Verification items for the finished model (mm, model axes). A direction names the side the tool comes from. Coordinates: 2 decimals unless noted, no trailing zeros. Write each loop counter-clockwise with the first axis right and the second up, starting at its lowest first coordinate (ties: lowest second). Pieces come first, ordered by that corner, then holes. Notation, with made-up numbers: (4.5, 57.5) -> (59.5, 57.5) arc R14 cw to (59.5, 78.5) -> close; hole circle Ø1 at (48, 68.25). An arc over 180 degrees is marked (long way). Answer in a Markdown table with one row per item.
```python
from build123d import *

# Parameters (mm, degrees)
F1_DEPTH      = 300
F1_DEPTH_BACK = 300


with BuildPart() as f1:
    # F0 (on Right) → F1 (new body, two sides)
    with BuildSketch(Plane.YZ) as f1_sk:
        with BuildLine():
            Line((110.183008, 157.357644), (5.9717, 8.528471))
            ThreePointArc((5.9717, 8.528471), (-1.176369, 2.259783), (-10.411341, 0))
            Line((-10.411341, 0), (-160.408616, 0))
            Line((-160.408616, 0), (-160.411341, -4))
            Line((-160.411341, -4), (-10.411341, -4))
            ThreePointArc((-10.411341, -4), (0.670626, -1.28826), (9.248308, 6.234166))
            Line((9.248308, 6.234166), (113.459616, 155.063338))
            ThreePointArc((113.459616, 155.063338), (147.770346, 185.15304), (192.098213, 196))
            Line((192.098213, 196), (231.673377, 196))
            ThreePointArc((231.673377, 196), (242.48282, 191.796437), (247.612492, 181.394492))
            Line((247.612492, 181.394492), (261.915687, 17.908216))
            ThreePointArc((261.915687, 17.908216), (269.610202, 2.305292), (285.824377, -4.000046))
            Line((285.824377, -4.000046), (339.588671, -4.000007))
            ThreePointArc((339.588671, -4.000007), (350.670628, -1.288263), (359.248303, 6.234158))
            Line((359.248303, 6.234158), (463.459616, 155.063338))
            ThreePointArc((463.459616, 155.063338), (497.770346, 185.15304), (542.098213, 196))
            Line((542.098213, 196), (581.673377, 196))
            ThreePointArc((581.673377, 196), (591.80723, 192.05916), (596.616297, 182.307336))
            Line((596.616297, 182.307336), (610.919489, 18.821106))
            ThreePointArc((610.919489, 18.821106), (618.613997, 3.218188), (634.828161, -3.087156))
            Line((634.828161, -3.087156), (688.592464, -3.087156))
            ThreePointArc((688.592464, -3.087156), (699.674431, -0.375416), (708.252113, 7.14701))
            Line((708.252113, 7.14701), (812.463422, 155.976182))
            ThreePointArc((812.463422, 155.976182), (846.774151, 186.065884), (891.102018, 196.912844))
            Line((891.102018, 196.912844), (930.677182, 196.912844))
            ThreePointArc((930.677182, 196.912844), (940.810305, 192.972673), (945.61993, 183.222154))
            Line((945.61993, 183.222154), (961.032927, -3.087156))
            Line((961.032927, -3.087156), (965.046592, -3.087156))
            Line((965.046592, -3.087156), (949.605558, 183.561051))
            ThreePointArc((949.605558, 183.561051), (943.516264, 195.918485), (930.677182, 200.912844))
            Line((930.677182, 200.912844), (891.102018, 200.912844))
            ThreePointArc((891.102018, 200.912844), (844.927157, 189.613928), (809.186814, 158.270488))
            Line((809.186814, 158.270488), (704.975505, 9.441316))
            ThreePointArc((704.975505, 9.441316), (697.827437, 3.172628), (688.592464, 0.912844))
            Line((688.592464, 0.912844), (634.828161, 0.912844))
            ThreePointArc((634.828161, 0.912844), (621.316357, 6.167298), (614.904268, 19.169729))
            Line((614.904268, 19.169729), (600.601076, 182.655959))
            ThreePointArc((600.601076, 182.655959), (594.50959, 195.008269), (581.673377, 200))
            Line((581.673377, 200), (542.098213, 200))
            ThreePointArc((542.098213, 200), (495.923351, 188.701083), (460.183008, 157.357644))
            Line((460.183008, 157.357644), (355.971695, 8.528464))
            ThreePointArc((355.971695, 8.528464), (348.823632, 2.259779), (339.588668, -7e-06))
            Line((339.588668, -7e-06), (285.824374, -4.6e-05))
            ThreePointArc((285.824374, -4.6e-05), (272.312561, 5.254403), (265.900466, 18.256839))
            Line((265.900466, 18.256839), (251.59727, 181.743115))
            ThreePointArc((251.59727, 181.743115), (245.185181, 194.745547), (231.673377, 200))
            Line((231.673377, 200), (192.098213, 200))
            ThreePointArc((192.098213, 200), (145.923351, 188.701083), (110.183008, 157.357644))
        make_face()
    extrude(amount=F1_DEPTH)
    extrude(f1_sk.sketch, amount=-F1_DEPTH_BACK)


solid = f1.part
```
1. Sectioned sample at D-D, the plane y = 407. Record the cut outline in (x, z).
Findings below:
| item | result |
|---|---|
| outline | (-300, 74.43) -> (300, 74.43) -> (300, 81.4) -> (-300, 81.4) -> close |
2. Sectioned sample at A-A, the plane z = 78. Record the cut outline in (x, y).
Findings below:
| item | result |
|---|---|
| outline | (-300, 54.62) -> (300, 54.62) -> (300, 59.5) -> (-300, 59.5) -> close; (-300, 256.66) -> (300, 256.66) -> (300, 260.67) -> (-300, 260.67) -> close; (-300, 404.62) -> (300, 404.62) -> (300, 409.5) -> (-300, 409.5) -> close; (-300, 605.74) -> (300, 605.74) -> (300, 609.76) -> (-300, 609.76) -> close; (-300, 752.98) -> (300, 752.98) -> (300, 757.86) -> (-300, 757.86) -> close; (-300, 954.32) -> (300, 954.32) -> (300, 958.34) -> (-300, 958.34) -> close |
3. Sectioned sample at C-C, the plane z = 170.5. Record the cut outline in (x, y).
Findings below:
| item | result |
|---|---|
| outline | (-300, 121.18) -> (300, 121.18) -> (300, 126.94) -> (-300, 126.94) -> close; (-300, 248.57) -> (300, 248.57) -> (300, 252.58) -> (-300, 252.58) -> close; (-300, 471.18) -> (300, 471.18) -> (300, 476.94) -> (-300, 476.94) -> close; (-300, 597.65) -> (300, 597.65) -> (300, 601.66) -> (-300, 601.66) -> close; (-300, 819.29) -> (300, 819.29) -> (300, 824.97) -> (-300, 824.97) -> close; (-300, 946.67) -> (300, 946.67) -> (300, 950.69) -> (-300, 950.69) -> close |
4. Go/stop test with flat-tipped pins: pin 1 (12 mm diameter, centred on x = 135, y = 904.5, fed in from -Z); pin 2 (6 mm diameter, centred on x = 226.5, y = 649, fed in from +Z); pin 3 (10 mm diameter, centred on x = 192, z = 104.5, fed in from -Y). Record where each tip stops, or that it passes through.
Findings below:
| item | result |
|---|---|
| pin 1 | stops at z = 196.91 |
| pin 2 | stops at z = 0.91 |
| pin 3 | stops at y = 69.67 |
5. Release check for a two-part mould opening along Y. For faces 6 (the face through (4.2, 957.434, 88.93)), 7 (the face through (4.2, 845.52, 189.92)), 8 (the face through (4, 212, 200)), 9 (the face through (4.2, 350.53, -1.36)) record: released by +Y, released by -Y, zero draft, split by the parting line, or undercut.
Findings below:
| item | result |
|---|---|
| face 6 | released by +Y |
| face 7 | undercut |
| face 8 | zero draft |
| face 9 | undercut |
6. Access from +Z, -Z, +X, -X, +Y, -Y to the whole of each face (thin tool, end or side, straight path). Record for faces 1 (the face through (4.2, 618.43, 3.39)), 2 (the face through (4, 661, -3.087)), 3 (the face through (4.2, 607.853, 99.768)), 4 (the face through (4, -84, 0)), 5 (the face through (300, 441, 129)).
Findings below:
| item | result |
|---|---|
| face 1 | -Z, +X, -X |
| face 2 | -Z, +X, -X, +Y |
| face 3 | +Z, +X, -X |
| face 4 | +Z, +X, -X, -Y |
| face 5 | +Z, -Z, +X, +Y, -Y |
7. Sectioned sample at B-B, the plane y = 562. Record the cut outline in (x, z).
Findings below:
| item | result |
|---|---|
| outline | (-300, 196) -> (300, 196) -> (300, 200) -> (-300, 200) -> close |
8. Material ranges on probe 1 along Y at (x, z) = (271, 23.5); probe 2 along Y at (x, z) = (99, 23); probe 3 along Z at (x, y) = (-0.5, 688), recorded low to high. Write a range as from..to.
Findings below:
| item | result |
|---|---|
| probe 1 | y = 16.45..21.34, 261.43..265.44, 366.45..371.34, 610.51..614.53, 714.82..719.7, 958.83..962.85 |
| probe 2 | y = 16.1..20.99, 261.47..265.49, 366.1..370.99, 610.55..614.57, 714.47..719.35, 958.87..962.89 |
| probe 3 | z = -3.09..0.91 |
